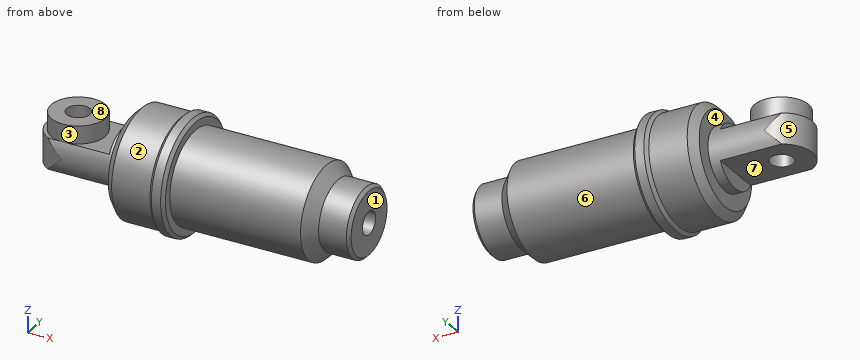
Autodesk Inventor part; units mm, degrees
ref_plane "YZ Plane" through (0, 0, 0) normal (1, 0, 0) x (0, 1, 0)
ref_plane "XZ Plane" through (0, 0, 0) normal (0, 1, 0) x (-1, 0, 0)
ref_plane "XY Plane" through (0, 0, 0) normal (0, 0, 1) x (1, 0, 0)
sketch "Sketch2" plane through (0, 0, 0) normal (0, 0, 1) x (1, 0, 0)
  line L0 (-6.1, 0) -> (36.6, 0) construction
  line L1 (0, -1.48) -> (0, 8.88) construction
  line L2 (0, 0) -> (0, 7)
  line L3 (0, 7) -> (6, 7)
  line L4 (6, 7) -> (6, 7.4)
  line L5 (6, 7.4) -> (8, 7.4)
  line L6 (8, 7.4) -> (8, 6)
  line L7 (8, 6) -> (26.5, 6)
  line L8 (26.5, 6) -> (26.5, 4.5)
  line L9 (26.5, 4.5) -> (30.5, 4.5)
  line L10 (30.5, 4.5) -> (30.5, 0)
  line L11 (0, 0) -> (30.5, 0)
  dimension "d0" = 14
  dimension "d1" = 30.5
  dimension "d2" = 8
  dimension "d3" = 14.8
  dimension "d4" = 9
  dimension "d5" = 4
  dimension "d6" = 12
  dimension "d7" = 6
revolve "Revolution1" add sketch "Sketch2" angle 360 about axis through (-10, 0, 0) along (1, 0, 0)
thread "Thread1"
chamfer "Chamfer1" distance 1.5 angle 45 1 edges at (26.5, -6, 0)
chamfer "Chamfer2" distance 0.4 angle 45 3 edges at (6, -7.4, 0) (8, -7.4, 0) (30.5, -4.5, 0)
chamfer "Chamfer3" distance 1 angle 45 1 edges at (0, -7, 0)
sketch "Sketch3" plane through (0, 0, 0) normal (-1, 0, 0) x (0, 0, 1)
  circle A0 centre (0, 0) radius 4
  dimension "d20" = 8
extrude "Extrusion1" add sketch "Sketch3" along normal blind 11.3
sketch "Sketch4" plane through (-11.3, 0, 0) normal (-1, 0, 0) x (0, 0, 1)
  line L0 (0, -10.36) -> (0, 10.36) construction
  circle A0 centre (0, 0) radius 4 construction
  circle A1 centre (0, 0) radius 4
  line L1 (-2, -3.4641) -> (-2, 3.4641)
  line L2 (2, 3.4641) -> (2, -3.4641)
  dimension "d23" = 4
extrude "Extrusion2" cut sketch "Sketch4" against normal blind 10 contours A1 L2 | L1 A1
sketch "Sketch5" plane through (-11.3, -3.4641, 2) normal (0, 0, 1) x (1, 0, 0)
  line L0 (-8.36, 3.4641) -> (50.16, 3.4641) construction
  circle A0 centre (4, 3.4641) radius 4
  line L1 (0, 0) -> (0, 6.9282) construction
  line L2 (10, 0) -> (0, 0) construction
  line L3 (10, 0) -> (10, 6.9282) construction
  line L4 (0, 6.9282) -> (10, 6.9282) construction
  line L5 (0, 0) -> (0, 6.9282) construction
  line L6 (11.3, 7.4641) -> (0, 7.4641) construction
  line L7 (11.3, -0.5359) -> (0, -0.5359) construction
  line L8 (4, -0.5359) -> (0, -0.5359)
  line L9 (0, -0.5359) -> (0, 7.4641)
  line L10 (0, 7.4641) -> (4, 7.4641)
  point P0 (11.3, 3.4641)
  point P1 (0, 3.4641)
  dimension "d26" = 8
extrude "Extrusion3" cut sketch "Sketch5" against normal through all contours A0 L9 L10 | L8 L9 A0
sketch "Sketch6" plane through (-1.3, -3.4641, 2) normal (0, 0, 1) x (1, 0, 0)
  arc A0 (-8, 6.9282) -> (-8, 0) centre (-6, 3.4641) ccw construction
  circle A1 centre (-6, 3.4641) radius 1.5
  point P0 (1.3, 3.4641)
  dimension "d29" = 3
extrude "Extrusion4" cut sketch "Sketch6" against normal through all
sketch "Sketch7" plane through (-1.3, -3.4641, 2) normal (0, 0, 1) x (1, 0, 0)
  circle A0 centre (-6, 3.4641) radius 1.5 construction
  circle A1 centre (-6, 3.4641) radius 1.5
  circle A2 centre (-6, 3.4641) radius 3.5
  point P0 (1.3, 3.4641)
  dimension "d32" = 7
extrude "Extrusion5" add sketch "Sketch7" along normal blind 2.3
sketch "Sketch8" plane through (30.5, 0, 0) normal (1, 0, 0) x (0, 0, -1)
  circle A0 centre (0, 0) radius 1.5
  dimension "d35" = 3
extrude "Extrusion6" cut sketch "Sketch8" against normal blind 20
properties part number "Corps" material "Aluminum 6061"
Can you work these out from the model? Positions are in its coordinate system, mm. Face numbers are marked on the shaded views. A direction names the side the tool comes from. Give positions to 0.01 mm unless a question says otherwise; leave off trailing zeros. Loops run counter-clockwise (first coordinate to the right, second up) from the corner with the lowest first, then second, coordinate; pieces in that order, holes last. Notation, with made-up numbers: M 73.25,-30.75 L 101.25,-30.75 A18 ccw 101.25,-11.75 Z; hole C 45.5,-10.75 d11. An arc over 180 degrees is marked long. Answer in a Markdown table with one row per item.
1. Which directions (+Z, -Z, +X, -X, +Y, -Y) give clear straight access to the entire face, cutting with the end or side of a thin tool? Please do the marked faces 4, 5, 6, 7 and 8.
Taken from the geometry:
| item | result |
|---|---|
| face 4 | none |
| face 5 | +Z, -Z, -X |
| face 6 | +X |
| face 7 | -Z, -X, +Y, -Y |
| face 8 | +Z, -X, +Y, -Y |
2. If I drill on line 1 along Z through (x, y) = (-2.5, 1.25); line 2 along X through (y, z) = (-3.25, -2.5); line 3 along Y through (x, z) = (-7.3, 0), over which ranges is the centre line in solid material (lowest first)?
Taken from the geometry:
| item | result |
|---|---|
| line 1 | z = -2 to 2 |
| line 2 | x = 0 to 30.5 |
| line 3 | y = -4 to -1.5, 1.5 to 4 |
3. Suppose I cut it at A-A on z = 2.75. Count the separate pieces of the cut face and the enclosed holes in it, plus the area to 3 significant figures.
Taken from the geometry:
| item | result |
|---|---|
| separate pieces | 2 |
| enclosed holes | 1 |
| area | 365 mm² |
4. Thinking about a two-plate mould opening in X: for the marked faces 1, 2 and 3, which applies, released by +X, released by -X, zero draft, split by the parting line, or undercut?
Taken from the geometry:
| item | result |
|---|---|
| face 1 | released by +X |
| face 2 | zero draft |
| face 3 | undercut |
5. For pin 1 Ø2.5 at (y, z) = (1, 0.5) entering from +X; pin 2 Ø5 at (x, y) = (-3, -1) entering from -Z; pin 3 Ø0.6 at (y, z) = (-1.5, -2.5) entering from -X; pin 4 Ø3 at (x, y) = (-10.5, -1) entering from +Z, each with a flat end and sliding along its axis, tell me the tip position at first contact or that it passes through.
Taken from the geometry:
| item | result |
|---|---|
| pin 1 | stops at x = 30.5 |
| pin 2 | stops at z = -4 |
| pin 3 | stops at x = -1.3 |
| pin 4 | stops at z = 4.3 |
6. Suppose I cut it at B-B on x = 5.5. Write out the boundary of the cut face in (y, z), plus the area to 3 significant figures.
Taken from the geometry:
| item | result |
|---|---|
| outline | C 0,0 d14 |
| area | 154 mm² |
